```python
from build123d import *

# Parameters (mm, degrees)
F0_W     = 105.41
F0_H     = 35.052
F0_R     = 1.9939
F1_DEPTH = 31.75
F2_W     = 105.41
F2_H     = 35.052
F3_DEPTH = 3.175
F4_R     = 3.81
F5_DEPTH = 25.4
F6_R     = 2.032
F7_DEPTH = 25.4


with BuildPart() as f1:
    # F0 (on Front) → F1 (new body)
    with BuildSketch(Plane.XZ):
        Rectangle(F0_W, F0_H)
        with Locations((-48.5902, -13.716)):
            Circle(F0_R, mode=Mode.SUBTRACT)
        with Locations((48.5902, -13.716)):
            Circle(F0_R, mode=Mode.SUBTRACT)
        with Locations((-48.5902, 13.716)):
            Circle(F0_R, mode=Mode.SUBTRACT)
        Polygon((-49.53, -8.662538), (-49.53, 8.662538), (-43.841538, 14.351), (43.841538, 14.351), (49.53, 8.662538), (49.53, -8.662538), (43.841538, -14.351), (-43.841538, -14.351), align=None, mode=Mode.SUBTRACT)
        with Locations((48.5902, 13.716)):
            Circle(F0_R, mode=Mode.SUBTRACT)
    extrude(amount=F1_DEPTH)

    # F2 (on face) → F3 (join)
    with BuildSketch(Plane(origin=(0, 0, 0), x_dir=(-1, 0, 0), z_dir=(0, 1, 0))):
        Rectangle(F2_W, F2_H)
    extrude(amount=-F3_DEPTH)

    # F4 (on face) → F5 (cut)
    with BuildSketch(Plane(origin=(0, 0, 0), x_dir=(-1, 0, 0), z_dir=(0, 1, 0))):
        with Locations((-38.1, -6.35)):
            Circle(F4_R)
        with Locations((38.1, -6.35)):
            Circle(F4_R)
    extrude(amount=-F5_DEPTH, mode=Mode.SUBTRACT)

    # F6 (on face) → F7 (cut)
    with BuildSketch(Plane.XZ.offset(3.175)):
        with Locations((22.225, 8.636)):
            Circle(F6_R)
        with Locations((-22.225, -8.636)):
            Circle(F6_R)
    extrude(amount=-F7_DEPTH, mode=Mode.SUBTRACT)


solid = f1.part
```
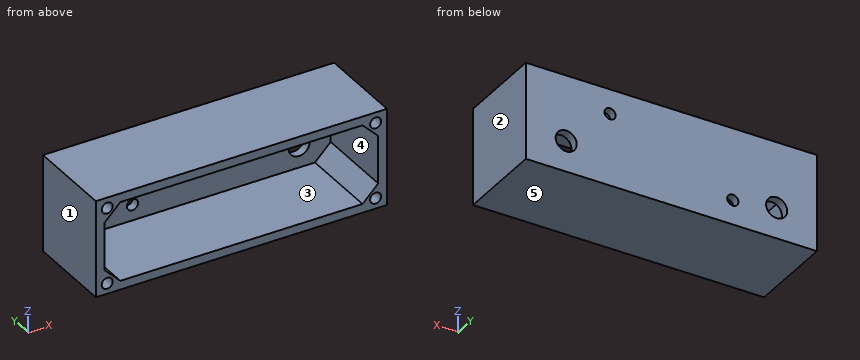
Here's how the part is built. I have some questions about the finished solid (model axes, mm). Face numbers are marked on the shaded views. A direction names the side the tool comes from. Give positions to 0.01 mm unless a question says otherwise; leave off trailing zeros. Loops run counter-clockwise (first coordinate to the right, second up) from the corner with the lowest first, then second, coordinate; pieces in that order, holes last. Notation, with made-up numbers: M -3.75,43.5 L 46.25,43.5 A20 cw 46.25,68.5 Z; hole C 65,15.5 d3. An arc over 180 degrees is marked long. Put each result on its own line as item: value. Start each with the question number.
(1) If we mould it in two halves opening along X, with no side actions, what happens to the marked faces 1, 2 and 3? For each: +X half, -X half, draft (parallel to the pull), parting line (faces both ways), or undercut.
(2) I want a section at B-B on y = -16. Please give me the cut outline in (x, z) (3 decimals).
(3) Will this pin go through, and if not, where does the flat tip stop? pin 1 Ø1.2 at (x, z) = (49, -14.5) entering from -Y (3 decimals).
(4) I want a section at A-A on x = -38.1. Please give me the cut outline in (y, z) (3 decimals).
(5) For the marked faces 4 and 5, which set-ups out of +Z, -Z, +X, -X, +Y, -Y let a thin tool reach every point of the face, with its end or its side?
(6) I need wall thicknesses on line 1 along Z through (x, y) = (7.5, -19.5); line 2 along X through (y, z) = (-1.5, -6) (3 decimals); line 3 along X through (y, z) = (-6, 4.5) (3 decimals). Which ranges of each line are inside material? Lowest first, please. Write a range as [from, to].
Answer block:
1. face 1: -X half
1. face 2: +X half
1. face 3: undercut
2. outline: M -52.705,-17.526 L 52.705,-17.526 L 52.705,17.526 L -52.705,17.526 Z; hole C -48.59,-13.716 d3.988; hole C -48.59,13.716 d3.988; hole M -49.53,-8.663 L -43.842,-14.351 L 43.842,-14.351 L 49.53,-8.663 L 49.53,8.663 L 43.842,14.351 L -43.842,14.351 L -49.53,8.663 Z; hole C 48.59,-13.716 d3.988; hole C 48.59,13.716 d3.988
3. pin 1: y = -3.175
4. outline: M -31.75,-17.526 L 0,-17.526 L 0,-10.16 L -3.175,-10.16 L -3.175,-14.351 L -31.75,-14.351 Z; M -31.75,14.351 L -3.175,14.351 L -3.175,-2.54 L 0,-2.54 L 0,17.526 L -31.75,17.526 Z
5. face 4: -Y
5. face 5: -Z, +X, -X, +Y, -Y
6. line 1: [-17.53, -14.35], [14.35, 17.53]
6. line 2: [-52.705, -41.894], [-34.306, 34.306], [41.894, 52.705]
6. line 3: [-52.705, -49.53], [49.53, 52.705]
